For this review, take the finished solid that the model builds, in its own axes (mm). A direction names the side the tool comes from. Give positions to 0.01 mm unless a question says otherwise; leave off trailing zeros. Loops run counter-clockwise (first coordinate to the right, second up) from the corner with the lowest first, then second, coordinate; pieces in that order, holes last. Notation, with made-up numbers: (53.25, 16) - (111.25, 16) arc R14 cw to (111.25, 27) - close; hole circle Ø9 at (37.5, -7). An arc over 180 degrees is marked (long way). Put each result on its own line as item: value.
from build123d import *

# Parameters (mm, degrees)
BOSS_EXTRU_1_DEPTH = 11
ESQUISSE2_R        = 5.5
BOSS_EXTRU_2_DEPTH = 5.8
ESQUISSE7_R        = 1
BOSS_EXTRU_3_DEPTH = 6


with BuildPart() as part:
    # Esquisse1 → Boss.-Extru.1 (new body)
    with BuildSketch(Plane(origin=(0, 0, 0), x_dir=(0, 0, -1), z_dir=(1, 0, 0))):
        Polygon((0, 17), (4.5, 17), (4.5, 20.43), (-27.5, 20.43), (-27.5, 17), (-23, 17), (-23, 0), (0, 0), align=None)
    extrude(amount=BOSS_EXTRU_1_DEPTH)

    # Esquisse2 → Boss.-Extru.2 (add)
    with BuildSketch(Plane(origin=(0, 20.43, 0), x_dir=(1, 0, 0), z_dir=(0, 1, 0))):
        with Locations((5.5, -5.6)):
            Circle(ESQUISSE2_R)
    extrude(amount=BOSS_EXTRU_2_DEPTH)

    # Esquisse7 → Boss.-Extru.3 (add)
    with BuildSketch(Plane(origin=(0, 26.23, 0), x_dir=(1, 0, 0), z_dir=(0, 1, 0))):
        with Locations((5.5, -5.6)):
            Circle(ESQUISSE7_R)
    extrude(amount=BOSS_EXTRU_3_DEPTH)


solid = part.part
1) Take a section at D-D on z = 16. State the section outline as (x, y) points, and give its area (3 significant figures).
Geometry check:
outline: (0, 0) - (11, 0) - (11, 20.43) - (0, 20.43) - close
area: 225 mm²
2) Take a section at B-B on z = 1. State the section outline as (x, y) points.
Geometry check:
outline: (0, 0) - (11, 0) - (11, 20.43) - (8.51, 20.43) - (8.51, 26.23) - (2.49, 26.23) - (2.49, 20.43) - (0, 20.43) - close
3) Wall thickness on line 1 (Z direction, x = 1.25, y = 4.5); line 2 (Y direction, x = 7, z = 15.5); line 3 (Y direction, x = 6.5, z = 4.5): over which ranges is each line inside the solid? List them lowest first.
Geometry check:
line 1: z = 0 to 23
line 2: y = 0 to 20.43
line 3: y = 0 to 26.23
4) Take a section at C-C on y = 10. State the section outline as (x, z) points.
Geometry check:
outline: (0, 0) - (11, 0) - (11, 23) - (0, 23) - close
5) Take a section at A-A on x = 5.5. State the section outline as (y, z) points.
Geometry check:
outline: (0, 0) - (17, 0) - (17, -4.5) - (20.43, -4.5) - (20.43, 0.1) - (26.23, 0.1) - (26.23, 4.6) - (32.23, 4.6) - (32.23, 6.6) - (26.23, 6.6) - (26.23, 11.1) - (20.43, 11.1) - (20.43, 27.5) - (17, 27.5) - (17, 23) - (0, 23) - close
6) Insertion check: pin 1 Ø3.5 at (x, z) = (6.5, 17) entering from +Y; pin 2 Ø5.5 at (x, y) = (6, 6) entering from +Z; pin 3 Ø5.5 at (x, y) = (6.5, 9) entering from -Z. Each pin has a flat end and moves straight along its axis. Give the tip position at first contact, or say it passes through.
Geometry check:
pin 1: stops at y = 20.43
pin 2: stops at z = 23
pin 3: stops at z = 0
7) For faces 1 (the face through (5, 8, 0)), 2 (the face through (8.457, 23.289, 0.962)), 3 (the face through (5, 17, 25)), list the 3-axis set-ups (+Z, -Z, +X, -X, +Y, -Y) from which the entire face can be reached by the end or side of a thin tool; tool diameter is ignored.
Geometry check:
face 1: -Z, +X, -X, -Y
face 2: +Y
face 3: +Z, +X, -X, -Y
